```python
from build123d import *

# Parameters (mm, degrees)
SKETCH1_R           = 0.25
BOSS_EXTRUDE1_DEPTH = 10
SKETCH2_R           = 0.5
BOSS_EXTRUDE2_DEPTH = 1
SCALE1_SCALE        = 100


with BuildPart() as part:
    # Sketch1 → Boss-Extrude1 (new body)
    with BuildSketch(Plane(origin=(0, 0, 0), x_dir=(1, 0, 0), z_dir=(0, 1, 0))):
        Circle(SKETCH1_R)
    extrude(amount=-BOSS_EXTRUDE1_DEPTH)

    # Sketch2 → Boss-Extrude2 (add)
    with BuildSketch(Plane.XZ.offset(10)):
        Circle(SKETCH2_R)
    extrude(amount=BOSS_EXTRUDE2_DEPTH)


with BuildPart() as part_1:
    # Scale1: scaled about (0, 0, 0)
    add(part.part.scale(SCALE1_SCALE))


solid = part_1.part
```
Model file for the job. Use its own axes, mm. A direction names the side the tool comes from. Give positions to 0.01 mm unless a question says otherwise; leave off trailing zeros. Order: outer loops, then holes, each group sorted by start corner. A loop starts at its lowest first (then second) coordinate and runs counter-clockwise, first axis right, second up.
1) Pin check, flat tips, straight feed: pin 1 (2 mm diameter, centred on y = -923.5, z = 0.5, fed in from -X); pin 2 (3 mm diameter, centred on y = -689.5, z = -27.5, fed in from +X); pin 3 (4 mm diameter, centred on y = -675.5, z = -12, fed in from -X); pin 4 (3 mm diameter, centred on x = 32.5, z = 12.5, fed in from +Y). Stop position of each tip, or through.
2) Saw through at B-B, the plane z = 0. Write the cut outline in (x, y), then the cut area to 3 significant figures.
3) Saw through at A-A, the plane x = 0. Write the cut outline in (y, z), then the cut area to 3 significant figures.
4) Mould opens along X. For faces 3 (the flat face through (10.4, -1000, 22.9)), 4 (the cylindrical face through (47.69, -1049.3, 15.02)) say: +X half, -X half, draft (parallel to the pull), parting line (faces both ways), or undercut.
5) Wall check: probe 1 along Y at (x, z) = (5, 45); probe 2 along X at (y, z) = (-478.5, -3.5); probe 3 along X at (y, z) = (-926, 1). Give the ranges that are in metal, low to high.
6) Saw through at C-C, the plane y = -631.5. Write the cut outline in (x, z), then the cut area to 3 significant figures.
7) 3-axis set-ups, long thin cutter, end or side, ignore diameter. For faces 1 (the flat face through (0, 0, 0)), 2 (the cylindrical face through (23.846, -493, -7.509)): which of +Z, -Z, +X, -X, +Y, -Y reach the whole face in a straight line?
8) Saw through at D-D, the plane x = -41. Write the cut outline in (y, z).
Computed:
1. pin 1: stops at x = -25
1. pin 2: passes through
1. pin 3: stops at x = -22.91
1. pin 4: stops at y = -1000
2. outline: (-50, -1100) - (50, -1100) - (50, -1000) - (25, -1000) - (25, 0) - (-25, 0) - (-25, -1000) - (-50, -1000) - close
2. area: 60,000 mm2
3. outline: (-1100, -50) - (-1000, -50) - (-1000, -25) - (0, -25) - (0, 25) - (-1000, 25) - (-1000, 50) - (-1100, 50) - close
3. area: 60,000 mm2
4. face 3: draft
4. face 4: parting line
5. probe 1: y = -1100 to -1000
5. probe 2: x = -24.75 to 24.75
5. probe 3: x = -24.98 to 24.98
6. outline: circle Ø50 at (0, 0)
6. area: 1,960 mm2
7. face 1: +Z, -Z, +X, -X, +Y
7. face 2: +Y
8. outline: (-1100, -28.62) - (-1000, -28.62) - (-1000, 28.62) - (-1100, 28.62) - close
